```python
from build123d import *

# Parameters (mm, degrees)
SKETCH_1_W                               = 92
SKETCH_1_H                               = 2
REAR_COVER_2MM_1_DEPTH                   = 65
SKETCH_3_W                               = 14
SKETCH_3_H                               = 6
DISPLAY_WIRE_EXIT_14X6_3_DEPTH           = 4
REAR_COVER_CAGE_ROOF_CLEARANCE_207_DEPTH = 94
SKETCH_5_R                               = 1.7
REAR_COVER_M3_CLEARANCE_FINAL_208_DEPTH  = 4


with BuildPart() as part:
    # Эскиз1 → Rear_cover_2mm_1 (new body)
    with BuildSketch(Plane.XY.offset(55)):
        with Locations((0, -45)):
            Rectangle(SKETCH_1_W, SKETCH_1_H)
    extrude(amount=REAR_COVER_2MM_1_DEPTH)

    # Эскиз3 → Display_wire_exit_14x6_3 (cut)
    with BuildSketch(Plane(origin=(0, -47, 0), x_dir=(1, 0, 0), z_dir=(0, 1, 0))):
        with Locations((0, -61)):
            Rectangle(SKETCH_3_W, SKETCH_3_H)
    extrude(amount=DISPLAY_WIRE_EXIT_14X6_3_DEPTH, mode=Mode.SUBTRACT)

    # Эскиз4 → Rear_cover_cage_roof_clearance_207 (cut)
    with BuildSketch(Plane(origin=(-47, 0, 0), x_dir=(0, 0, -1), z_dir=(1, 0, 0))):
        Polygon((-10, -47), (-10, -40), (-57.861284772, -40), (-55.985640425, -47), align=None)
    extrude(amount=REAR_COVER_CAGE_ROOF_CLEARANCE_207_DEPTH, mode=Mode.SUBTRACT)

    # Эскиз5 → Rear_cover_M3_clearance_final_208 (cut)
    with BuildSketch(Plane(origin=(0, -47, 0), x_dir=(1, 0, 0), z_dir=(0, 1, 0))):
        with Locations(Location((-41, -62, 0), (0, 0, 90))):
            Circle(SKETCH_5_R)
        with Locations(Location((41, -62, 0), (0, 0, 90))):
            Circle(SKETCH_5_R)
        with Locations(Location((-41, -115, 0), (0, 0, 90))):
            Circle(SKETCH_5_R)
        with Locations(Location((41, -115, 0), (0, 0, 90))):
            Circle(SKETCH_5_R)
    extrude(amount=REAR_COVER_M3_CLEARANCE_FINAL_208_DEPTH, mode=Mode.SUBTRACT)


solid = part.part
```
The model under review builds one solid part; all positions refer to its coordinate system, in mm. A direction names the side the tool comes from. Round coordinates to 2 decimals unless told otherwise and drop trailing zeros. Order: outer loops, then holes, each group sorted by start corner. A loop starts at its lowest first (then second) coordinate and runs counter-clockwise, first axis right, second up. Notation, with made-up numbers: (68, 58) -> (78, 58) arc R14 ccw to (78, 75) -> close; hole circle Ø9 at (10, -37.5). An arc over 180 degrees is marked (long way). Use a Markdown table: item, result.
Q1. Mouldability with a two-part tool opening along X and no side actions: class faces 1 (the flat face through (-46, -45, 88)), 2 (the flat face through (0, -45, 58)), 3 (the flat face through (-1, -46, 88)) as +X half, -X half, draft (parallel to the pull), parting line (faces both ways), or undercut.
Values:
| item | result |
|---|---|
| face 1 | -X half |
| face 2 | undercut |
| face 3 | draft |
Q2. We need section D-D on z = 115. Write out the cut boundary in (x, y), then the cut area to 3 significant figures.
Values:
| item | result |
|---|---|
| outline | (-46, -46) -> (-42.7, -46) -> (-42.7, -44) -> (-46, -44) -> close; (-39.3, -46) -> (39.3, -46) -> (39.3, -44) -> (-39.3, -44) -> close; (42.7, -46) -> (46, -46) -> (46, -44) -> (42.7, -44) -> close |
| area | 170 mm^2 |
Q3. For line 1 (X direction, y = -44.75, z = 115); line 2 (X direction, y = -44.5, z = 62); line 3 (X direction, y = -44.5, z = 114.5), list the stretches that pass through material, from the lowest coordinate up.
Values:
| item | result |
|---|---|
| line 1 | x = -46 to -42.7, -39.3 to 39.3, 42.7 to 46 |
| line 2 | x = -46 to -42.7, -39.3 to -7, 7 to 39.3, 42.7 to 46 |
| line 3 | x = -46 to -42.62, -39.38 to 39.38, 42.62 to 46 |
Q4. We need section B-B on z = 62. Write out the cut boundary in (x, y), then the cut area to 3 significant figures.
Values:
| item | result |
|---|---|
| outline | (-46, -46) -> (-42.7, -46) -> (-42.7, -44) -> (-46, -44) -> close; (-39.3, -46) -> (-7, -46) -> (-7, -44) -> (-39.3, -44) -> close; (7, -46) -> (39.3, -46) -> (39.3, -44) -> (7, -44) -> close; (42.7, -46) -> (46, -46) -> (46, -44) -> (42.7, -44) -> close |
| area | 142 mm^2 |
Q5. We need section A-A on x = -41. Write out the cut boundary in (y, z).
Values:
| item | result |
|---|---|
| outline | (-46, 56.25) -> (-44, 56.79) -> (-44, 60.3) -> (-46, 60.3) -> close; (-46, 63.7) -> (-44, 63.7) -> (-44, 113.3) -> (-46, 113.3) -> close; (-46, 116.7) -> (-44, 116.7) -> (-44, 120) -> (-46, 120) -> close |
Q6. We need section C-C on x = 2.5. Write out the cut boundary in (y, z).
Values:
| item | result |
|---|---|
| outline | (-46, 56.25) -> (-44, 56.79) -> (-44, 58) -> (-46, 58) -> close; (-46, 64) -> (-44, 64) -> (-44, 120) -> (-46, 120) -> close |
Q7. Tool access review of faces 4 (the flat face through (-0.644, -44.986, 56.525)), 5 (the flat face through (0, -45, 64)): name each direction out of +Z, -Z, +X, -X, +Y, -Y from which nothing blocks a thin tool from reaching the whole face with its end or side.
Values:
| item | result |
|---|---|
| face 4 | -Z, +X, -X, +Y |
| face 5 | +Y, -Y |
